Here's how the part is built. I have some questions about the finished solid (model axes, mm). A direction names the side the tool comes from. Coordinates: 2 decimals unless noted, no trailing zeros. Order: outer loops, then holes, each group sorted by start corner. A loop starts at its lowest first (then second) coordinate and runs counter-clockwise, first axis right, second up. Notation, with made-up numbers: (73.5, -12.5) - (85.5, -12.5) arc R4 ccw to (85.5, -7.5) - close; hole circle Ø8 at (72, -17.75). An arc over 180 degrees is marked (long way). Answer as CSV lines item,"result". Start each with the question number.
Item 1: On a 3-axis mill with a long thin cutter (end or side, diameter ignored), from which of +Z, -Z, +X, -X, +Y, -Y can I reach the whole of each face in a straight line? I mean faces 4 (the face through (11.22, -11.96, 8.96)), 5 (the face through (15, -3, 9)), 6 (the face through (0.78, -11.96, 3.04)), 7 (the face through (27.99, 1.19, 11.37)). Say none if no direction works.
Item 2: I need wall thicknesses on line 1 (X direction, y = 19, z = 10.25); line 2 (X direction, y = -4, z = 8.5); line 3 (X direction, y = -2.5, z = 4.25). Which ranges of each line are inside material? Lowest first, please.
Item 3: I'm going to push flat-ended pins straight in: pin 1 (6 mm diameter, centred on x = 22.5, z = 3.5, fed in from +Y); pin 2 (6 mm diameter, centred on y = 2.5, z = 4, fed in from -X); pin 3 (6 mm diameter, centred on x = 12.5, y = 13.5, fed in from -Z). Where does each tip first touch, or does it pass through?
Item 4: Imagine slicing it at A-A on y = -8.5. List the corners of the cut face in (x, z) for me.
Item 5: We'd pull the mould along Y, two halves only. Please class faces 1 (the face through (10.9, -21, 7.6)), 2 (the face through (18, 0, 12)), 3 (the face through (17.96, 5.22, 8.96)): pulls with the +Y half, pulls with the -Y half, needs draft (parallel to the pull), parting line crosses it, or undercut.
from build123d import *

# Parameters (mm, degrees)
SZKIC1_W                    = 12
SZKIC1_H                    = 12
DODANIE_WYCI_GNI_CIE1_DEPTH = 12
SZKIC2_R                    = 5.5
DODANIE_WYCI_GNI_CIE2_DEPTH = 1
SZKIC3_R                    = 4
DODANIE_WYCI_GNI_CIE3_DEPTH = 2
SZKIC4_R                    = 4
DODANIE_WYCI_GNI_CIE4_DEPTH = 6
SZKIC7_R                    = 5.5
DODANIE_WYCI_GNI_CIE5_DEPTH = 2
SZKIC8_R                    = 5.5
DODANIE_WYCI_GNI_CIE6_DEPTH = 1
SZKIC9_R                    = 4
DODANIE_WYCI_GNI_CIE7_DEPTH = 2
DODANIE_WYCI_GNI_CIE8_DEPTH = 6
SZKIC13_R                   = 5.5
DODANIE_WYCI_GNI_CIE9_DEPTH = 2


with BuildPart() as part:
    # Szkic1 → Dodanie-wyciągnięcie1 (new body)
    with BuildSketch(Plane.XY):
        with Locations((6, 0)):
            Rectangle(SZKIC1_W, SZKIC1_H)
    extrude(amount=DODANIE_WYCI_GNI_CIE1_DEPTH)

    # Szkic2 → Dodanie-wyciągnięcie2 (add)
    with BuildSketch(Plane.XZ.offset(6)):
        with Locations(Location((6, 6, 0), (0, 0, 90))):
            Circle(SZKIC2_R)
    dodanie_wyci_gni_cie2 = extrude(amount=DODANIE_WYCI_GNI_CIE2_DEPTH)

    # Szkic3 → Dodanie-wyciągnięcie3 (add)
    with BuildSketch(Plane.XZ.offset(7)):
        with Locations(Location((6, 6, 0), (0, 0, 270))):
            Circle(SZKIC3_R)
    dodanie_wyci_gni_cie3 = extrude(amount=DODANIE_WYCI_GNI_CIE3_DEPTH)

    # Szkic4 → Dodanie-wyciągnięcie4 (add)
    with BuildSketch(Plane.XZ.offset(9)):
        Polygon((9.464101615, 0), (12.92820323, 6), (9.464101615, 12), (2.535898385, 12), (-0.92820323, 6), (2.535898385, 0), align=None)
        with Locations(Location((6, 6, 0), (0, 0, 270))):
            Circle(SZKIC4_R, mode=Mode.SUBTRACT)
        with Locations(Location((6, 6, 0), (0, 0, 270))):
            Circle(SZKIC4_R)
    dodanie_wyci_gni_cie4 = extrude(amount=DODANIE_WYCI_GNI_CIE4_DEPTH)

    # Szkic5 for Wyci_gni_cie → Wyciągnięcie po profilach1 section 0
    with BuildSketch(Plane(origin=(0, -21, 0), x_dir=(-1, 0, 0), z_dir=(0, -1, 0))):
        with BuildLine():
            # circular arc as an exact rational Bezier (weights 1, cos(half-angle), 1)
            Bezier((-8.5, -1.669872981), (-11, -3.113248654), (-11, -6), weights=[1, 0.866025404, 1])
            Bezier((-11, -6), (-11, -8.886751346), (-8.5, -10.330127019), weights=[1, 0.866025404, 1])
            Bezier((-8.5, -10.330127019), (-6, -11.773502692), (-3.5, -10.330127019), weights=[1, 0.866025404, 1])
            Bezier((-3.5, -10.330127019), (-1, -8.886751346), (-1, -6), weights=[1, 0.866025404, 1])
            Bezier((-1, -6), (-1, -3.113248654), (-3.5, -1.669872981), weights=[1, 0.866025404, 1])
            Bezier((-3.5, -1.669872981), (-6, -0.226497308), (-8.5, -1.669872981), weights=[1, 0.866025404, 1])
        make_face()
    # Szkic6 → Wyciągnięcie po profilach1 section 1
    with BuildSketch(Plane.XZ.offset(15)):
        Polygon((9.464101615, 0), (12.92820323, 6), (9.464101615, 12), (2.535898385, 12), (-0.92820323, 6), (2.535898385, 0), align=None)
    wyci_gni_cie_po_profilach1 = loft()

    # Szkic7 → Dodanie-wyciągnięcie5 (add)
    with BuildSketch(Plane.XZ.offset(21)):
        with Locations(Location((6, 6, 0), (0, 0, 90))):
            Circle(SZKIC7_R)
    dodanie_wyci_gni_cie5 = extrude(amount=DODANIE_WYCI_GNI_CIE5_DEPTH)

    # Lustro1: Dodanie-wyciągnięcie2, Dodanie-wyciągnięcie3, Dodanie-wyciągnięcie4, Wyciągnięcie po profilach1, Dodanie-wyciągnięcie5 across plane
    add(dodanie_wyci_gni_cie2.mirror(Plane.ZX))
    add(dodanie_wyci_gni_cie3.mirror(Plane.ZX))
    add(dodanie_wyci_gni_cie4.mirror(Plane.ZX))
    add(wyci_gni_cie_po_profilach1.mirror(Plane.ZX))
    add(dodanie_wyci_gni_cie5.mirror(Plane.ZX))

    # Szkic8 → Dodanie-wyciągnięcie6 (add)
    with BuildSketch(Plane(origin=(12, 0, 0), x_dir=(0, 0, -1), z_dir=(1, 0, 0))):
        with Locations(Location((-6, 0, 0), (0, 0, 270))):
            Circle(SZKIC8_R)
    extrude(amount=DODANIE_WYCI_GNI_CIE6_DEPTH)

    # Szkic9 → Dodanie-wyciągnięcie7 (add)
    with BuildSketch(Plane(origin=(13, 0, 0), x_dir=(0, 0, -1), z_dir=(1, 0, 0))):
        with Locations(Location((-6, 0, 0), (0, 0, 90))):
            Circle(SZKIC9_R)
    extrude(amount=DODANIE_WYCI_GNI_CIE7_DEPTH)

    # Szkic10 → Dodanie-wyciągnięcie8 (add)
    with BuildSketch(Plane(origin=(15, 0, 0), x_dir=(0, 0, -1), z_dir=(1, 0, 0))):
        Polygon((-6, 6.92820323), (-12, 3.464101615), (-12, -3.464101615), (-6, -6.92820323), (0, -3.464101615), (0, 3.464101615), align=None)
    extrude(amount=DODANIE_WYCI_GNI_CIE8_DEPTH)

    # Szkic12 → Wyciągnięcie po profilach2 section 0
    with BuildSketch(Plane(origin=(21, 0, 0), x_dir=(0, 0, -1), z_dir=(1, 0, 0))):
        Polygon((0, 3.464101615), (-6, 6.92820323), (-12, 3.464101615), (-12, -3.464101615), (-6, -6.92820323), (0, -3.464101615), align=None)
    # Szkic11 for Wyci_gni_cie → Wyciągnięcie po profilach2 section 1
    with BuildSketch(Plane(origin=(27, 0, 0), x_dir=(0, 0, -1), z_dir=(1, 0, 0))):
        with BuildLine():
            Bezier((-1.669872981, 2.5), (-3.113248654, 5), (-6, 5), weights=[1, 0.866025404, 1])
            Bezier((-6, 5), (-8.886751346, 5), (-10.330127019, 2.5), weights=[1, 0.866025404, 1])
            Bezier((-10.330127019, 2.5), (-11.773502692, 0), (-10.330127019, -2.5), weights=[1, 0.866025404, 1])
            Bezier((-10.330127019, -2.5), (-8.886751346, -5), (-6, -5), weights=[1, 0.866025404, 1])
            Bezier((-6, -5), (-3.113248654, -5), (-1.669872981, -2.5), weights=[1, 0.866025404, 1])
            Bezier((-1.669872981, -2.5), (-0.226497308, 0), (-1.669872981, 2.5), weights=[1, 0.866025404, 1])
        make_face()
    loft()

    # Szkic13 → Dodanie-wyciągnięcie9 (add)
    with BuildSketch(Plane(origin=(27, 0, 0), x_dir=(0, 0, -1), z_dir=(1, 0, 0))):
        with Locations(Location((-6, 0, 0), (0, 0, 270))):
            Circle(SZKIC13_R)
    extrude(amount=DODANIE_WYCI_GNI_CIE9_DEPTH)


solid = part.part
Responses:
1,face 4,"+Z, +X, -Y"
1,face 5,"none"
1,face 6,"-Z, -X, -Y"
1,face 7,"+X"
2,line 1,"x = 2.54 to 9.46"
2,line 2,"x = 0 to 13, 15 to 29"
2,line 3,"x = 0 to 29"
3,pin 1,"stops at y = 6.93"
3,pin 2,"stops at x = 0"
3,pin 3,"stops at z = 0.06"
4,outline,"circle Ø8 at (6, 6)"
5,face 1,"undercut"
5,face 2,"needs draft"
5,face 3,"pulls with the +Y half"
